The listing builds one solid part. Answer for the finished solid, in the listing's coordinates (mm). Face numbers are marked on the shaded views. A direction names the side the tool comes from. Give positions to 0.01 mm unless a question says otherwise; leave off trailing zeros. Write each loop counter-clockwise with the first axis right and the second up, starting at its lowest first coordinate (ties: lowest second). Pieces come first, ordered by that corner, then holes. Notation, with made-up numbers: (6.25, 76) -> (62.25, 76) arc R31 cw to (62.25, 112) -> close; hole circle Ø1 at (-2, -19.75). An arc over 180 degrees is marked (long way). One line per question, with ' | ' between items.
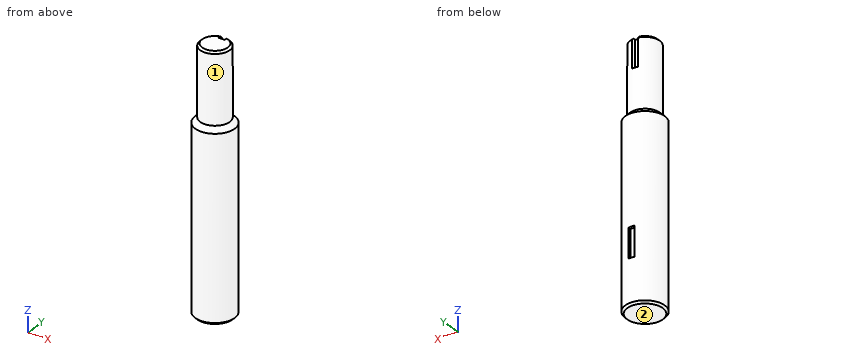
from build123d import *

# Parameters (mm, degrees)
CHAMFER1_SIZE      = 1
SKETCH3_W          = 3.25
SKETCH3_H          = 3.25
CUT_EXTRUDE2_DEPTH = 15
SKETCH4_W          = 3.25
SKETCH4_H          = 3.25
CUT_EXTRUDE3_DEPTH = 15
CHAMFER2_SIZE      = 3


with BuildPart() as part:
    # Sketch1 → Revolve1 (revolve)
    with BuildSketch(Plane(origin=(0, 0, 0), x_dir=(1, 0, 0), z_dir=(0, 1, 0)), mode=Mode.PRIVATE) as revolve1_sk:
        Polygon((10, 35), (7.5, 35), (7.5, 0), (0, 0), (0, 130), (10, 130), align=None)
    revolve(revolve1_sk.sketch.rotate(Axis((0, 0, -130), (0, 0, 1)), 180), axis=Axis((0, 0, -130), (0, 0, 1)))

    # Chamfer1
    chamfer1_edges = [part.edges().sort_by_distance(p)[0] for p in [
        (7.5, 0, 0),
        (10, 0, -130),
    ]]
    chamfer(chamfer1_edges, length=CHAMFER1_SIZE)

    # Sketch3 → Cut-Extrude2 (cut)
    with BuildSketch(Plane(origin=(0, 0, -107.5), x_dir=(-1, 0, 0), z_dir=(0, 0, -1))):
        with Locations((0, 10)):
            Rectangle(SKETCH3_W, SKETCH3_H)
    extrude(amount=-CUT_EXTRUDE2_DEPTH, mode=Mode.SUBTRACT)

    # Sketch4 → Cut-Extrude3 (cut)
    with BuildSketch(Plane.XY):
        with Locations((0, 6.5)):
            Rectangle(SKETCH4_W, SKETCH4_H)
    extrude(amount=-CUT_EXTRUDE3_DEPTH, mode=Mode.SUBTRACT)

    # Chamfer2
    # the kernel refuses this chamfer: 3 mm, written as the material it takes off along each edge
    with BuildSketch(Plane(origin=(0, 0, -35), x_dir=(-1, 0, 0), z_dir=(0, 1, 0))) as chamfer2_piece_1_section:
        Polygon((10 - CHAMFER2_SIZE, 0), (10, -CHAMFER2_SIZE), (10, 0), align=None)
    chamfer2_piece_1 = revolve(axis=Axis((0, 0, -35), (0, 0, 1)), mode=Mode.PRIVATE)
    chamfer2_piece_1 = chamfer2_piece_1 - Plane(origin=(0, 0, -36.746638668), x_dir=(-1, 0, 0), z_dir=(0, 0, 1)) * Cylinder(7.5, 41, mode=Mode.PRIVATE)
    add(chamfer2_piece_1, mode=Mode.SUBTRACT)


solid = part.part
Item 1: Find section B-B (x = 0). Write down the section's boundary in (y, z) (3 decimals).
Answers below:
outline: (-10, -129) -> (-9, -130) -> (9, -130) -> (10, -129) -> (10, -107.5) -> (8.375, -107.5) -> (8.375, -92.5) -> (10, -92.5) -> (10, -38) -> (7.5, -35.5) -> (7.5, -15) -> (4.875, -15) -> (4.875, 0) -> (-6.5, 0) -> (-7.5, -1) -> (-7.5, -35.5) -> (-10, -38) -> close
Item 2: Flat-ended cylindrical pins translate along their axes: pin 1 (1.6 mm diameter, centred on y = 9, z = -102, fed in from +X); pin 2 (2.5 mm diameter, centred on y = 5.5, z = -5.5, fed in from +X); pin 3 (5 mm diameter, centred on x = 7.5, z = -94.5, fed in from -Y). Find the tip coordinate at first contact, or state that the pin passes through.
Answers below:
pin 1: x = 5.72 | pin 2: x = 6.18 | pin 3: y = -8.66
Item 3: Find section D-D (z = -17). Write down the section's boundary in (x, y).
Answers below:
outline: circle Ø15 at (0, 0)
Item 4: Find section A-A (y = 0). Write down the section's boundary in (x, z).
Answers below:
outline: (-10, -129) -> (-9, -130) -> (9, -130) -> (10, -129) -> (10, -38) -> (7.5, -35.5) -> (7.5, -1) -> (6.5, 0) -> (-6.5, 0) -> (-7.5, -1) -> (-7.5, -35.5) -> (-10, -38) -> close
Item 5: Find section C-C (z = -94.5). Write down the section's boundary in (x, y) (3 decimals), then the cut area to 3 significant figures.
Answers below:
outline: (-1.625, 8.375) -> (-1.625, 9.867) arc R10 ccw (long way) to (1.625, 9.867) -> (1.625, 8.375) -> close | area: 309 mm²
Item 6: A tool of negligible diameter and unlimited length cuts with its end or side. For the marked faces 1 and 2, from which of +Z, -Z, +X, -X, +Y, -Y can it reach the whole face along a straight path? Write none if from no direction.
Answers below:
face 1: +Z | face 2: -Z, +X, -X, +Y, -Y
Item 7: Consider line 1 (Z direction, x = 0.25, y = 5); line 2 (Y direction, x = 0.75, z = -86.5); line 3 (Z direction, x = 3, y = 7). Determine where each line is inside the solid, lowest interval first. Write a range as [from, to].
Answers below:
line 1: [-130, -15] | line 2: [-9.97, 9.97] | line 3: [-130, -35.62]
